```python
from build123d import *

# Parameters (mm, degrees)
F0_W     = 41
F0_H     = 41
F0_R     = 11
F1_DEPTH = 41
F2_W     = 6
F2_H     = 11.5
F3_DEPTH = 41.001
F4_R     = 2.5
F5_DEPTH = 41.001


# Not quite as in the source:
# - a feature names something its author has since deleted; it is built from what else it names


with BuildPart() as f1:
    # F0 (on Front) → F1 (new body)
    with BuildSketch(Plane.XZ):
        Rectangle(F0_W, F0_H)
        Circle(F0_R, mode=Mode.SUBTRACT)
    extrude(amount=F1_DEPTH)

    # F2 (on Front) → F3 (cut, through all)
    with BuildSketch(Plane.XZ):
        with Locations((0, -14.9551387876)):
            Rectangle(F2_W, F2_H)
    extrude(amount=F3_DEPTH, mode=Mode.SUBTRACT)

    # F4 (on face) → F5 (cut, through all)
    with BuildSketch(Plane.YZ.offset(20.5)):
        with Locations((-31, -15)):
            Circle(F4_R)
        with Locations((-10, -15)):
            Circle(F4_R)
    extrude(amount=-F5_DEPTH, mode=Mode.SUBTRACT)


solid = f1.part
```
CAD build for the part. Positions are in the model's coordinates, mm. A direction names the side the tool comes from. Coordinates: 2 decimals unless noted, no trailing zeros. Order: outer loops, then holes, each group sorted by start corner. A loop starts at its lowest first (then second) coordinate and runs counter-clockwise, first axis right, second up. Notation, with made-up numbers: M 19.5,23.5 L 50.5,23.5 A17 ccw 50.5,32.5 Z; hole C 18,21 d4. An arc over 180 degrees is marked long. Write each question's results on one line, items separated by ' | '. Start each with the question number.
Q1. Which spindle directions (+Z, -Z, +X, -X, +Y, -Y) get a long thin tool onto all of the face, cutting with end or side? Do faces 1 (the flat face through (-3, -20, -16)), 2 (the flat face through (0, -20, 20.5)). Say none if no direction does.
Q2. Cut at A-A (y = -31). List the corners of the cut face in (x, z).
Q3. Flat gauge pin, fed straight in: P1, Ø4.5, axis at y = -31, z = -15, coming from the -X side. Where does the tip first touch, or does it go through?
Q4. Cut at C-C (x = -8). List the corners of the cut face in (y, z).
Q5. Cut at D-D (z = 0). List the corners of the cut face in (x, y).
Q6. Drill centre lines: probe 1 along X at (y, z) = (-6, -17); probe 2 along X at (y, z) = (-30, 0); probe 3 along Z at (x, y) = (-10, -31). Where is each one in solid material? Low to high. Write a range as from..to.
Q7. Cut at B-B (z = -15). List the corners of the cut face in (x, y), then the cut area to 4 significant figures.
Q8. Pull direction Y, two halves, no side cores. Call faces 3 (the flat face through (20.5, -20, 0)), 4 (the cylindrical face through (-11.6, -33.5, -14.9)), 5 (the flat face through (-9, 0, 9)): +Y half, -Y half, draft (parallel to the pull), parting line (faces both ways), or undercut.
Found:
1) face 1: -Z, +Y, -Y | face 2: +Z, +X, -X, +Y, -Y
2) outline: M -20.5,-20.5 L -3,-20.5 L -3,-17.5 L -20.5,-17.5 Z; M -20.5,-12.5 L -3,-12.5 L -3,-10.58 A11 cw long 3,-10.58 L 3,-12.5 L 20.5,-12.5 L 20.5,20.5 L -20.5,20.5 Z; M 3,-20.5 L 20.5,-20.5 L 20.5,-17.5 L 3,-17.5 Z
3) P1: through
4) outline: M -41,-20.5 L 0,-20.5 L 0,-7.55 L -41,-7.55 Z; M -41,7.55 L 0,7.55 L 0,20.5 L -41,20.5 Z; hole C -31,-15 d5; hole C -10,-15 d5
5) outline: M -20.5,-41 L -11,-41 L -11,0 L -20.5,0 Z; M 11,-41 L 20.5,-41 L 20.5,0 L 11,0 Z
6) probe 1: -20.5..-3, 3..20.5 | probe 2: -20.5..-11, 11..20.5 | probe 3: -20.5..-17.5, -12.5..-4.58, 4.58..20.5
7) outline: M -20.5,-41 L -3,-41 L -3,-33.5 L -20.5,-33.5 Z; M -20.5,-28.5 L -3,-28.5 L -3,-12.5 L -20.5,-12.5 Z; M -20.5,-7.5 L -3,-7.5 L -3,0 L -20.5,0 Z; M 3,-41 L 20.5,-41 L 20.5,-33.5 L 3,-33.5 Z; M 3,-28.5 L 20.5,-28.5 L 20.5,-12.5 L 3,-12.5 Z; M 3,-7.5 L 20.5,-7.5 L 20.5,0 L 3,0 Z | area: 1,085 mm²
8) face 3: draft | face 4: undercut | face 5: +Y half
